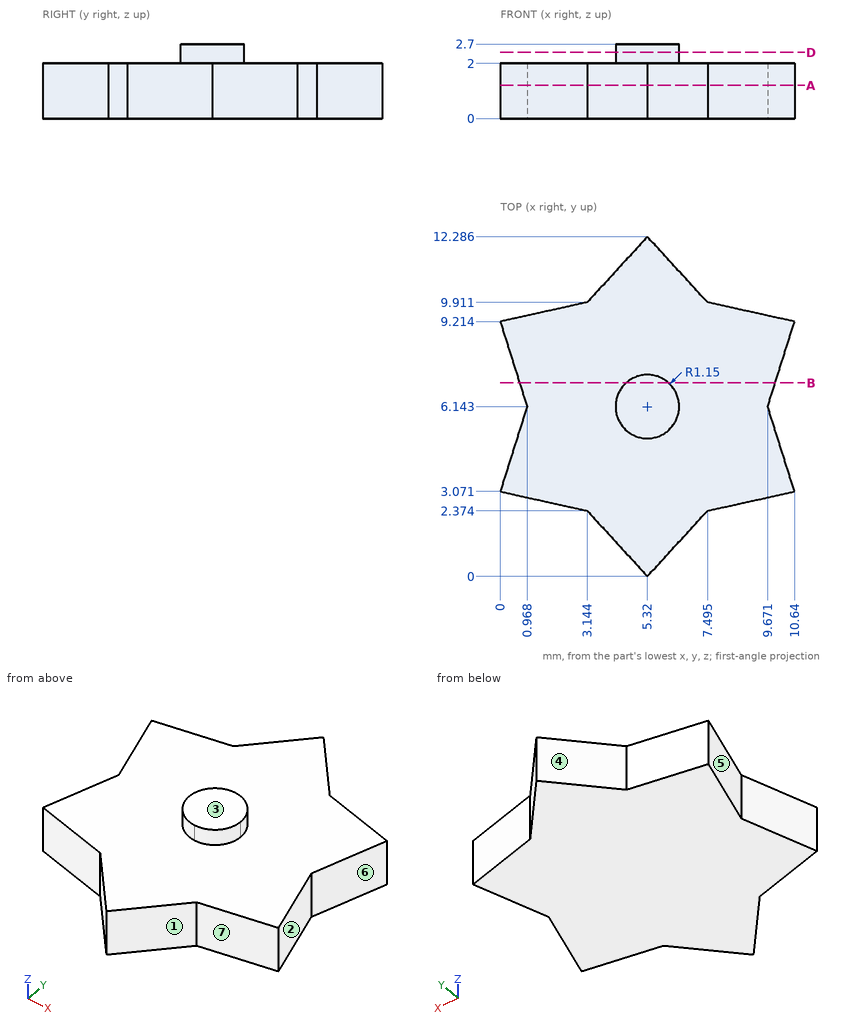
Part print with two shaded views. Sizes in mm from the minimum x, y, z corner. A direction names the side the tool comes from. Round coordinates to 2 decimals unless told otherwise and drop trailing zeros. Order: outer loops, then holes, each group sorted by start corner. A loop starts at its lowest first (then second) coordinate and runs counter-clockwise, first axis right, second up. Notation, with made-up numbers: M 40,-34.75 L 77,-34.75 A28 ccw 77,-1.75 Z; hole C 53,14 d7. An arc over 180 degrees is marked long. Answer in a Markdown table with one row per item. Add a question column.
Q1. Wall check: L1, parallel to Z at x = 5.75, y = 7.5; L2, parallel to X at y = 3.25, z = 1.2 (1 decimal); L3, parallel to Y at x = 6.25, z = 1.8 (1 decimal). Give the ranges that are in metal, low to high. Write a range as from..to.
Q2. Cut at B-B on y = 7. Give the cut face in (x, z).
Q3. Cut at D-D on z = 2.4. Give the cut face in (x, y).
Q4. 3-axis set-ups, long thin cutter, end or side, ignore diameter. For the marked faces 5, 6 and 7: which of +Z, -Z, +X, -X, +Y, -Y reach the whole face in a straight line?
Q5. Cut at A-A on z = 1.2. Give the cut face in (x, y) (1 decimal).
Q6. Mould opens along Y. For the marked faces 1, 2, 3 and 4 say: +Y half, -Y half, draft (parallel to the pull), parting line (faces both ways), or undercut.
Q7. Pin check, flat tip, straight feed: pin 1 (4 mm diameter, centred on x = 2, y = 4.5, fed in from +Z). Stop position of the tip, or through.
Established:
| question | item | result |
|---|---|---|
| 1 | L1 | z = 0..2 |
| 1 | L2 | x = 0.1..10.6 |
| 1 | L3 | y = 1..11.3 |
| 2 | outline | M 0.7,0 L 9.94,0 L 9.94,2 L 6.09,2 L 6.09,2.7 L 4.55,2.7 L 4.55,2 L 0.7,2 Z |
| 3 | outline | C 5.32,6.14 d2.3 |
| 4 | face 5 | +Z, -Z, -X |
| 4 | face 6 | +Z, -Z, +X |
| 4 | face 7 | +Z, -Z, +X, -Y |
| 5 | outline | M 0,3.1 L 3.1,2.4 L 5.3,0 L 7.5,2.4 L 10.6,3.1 L 9.7,6.1 L 10.6,9.2 L 7.5,9.9 L 5.3,12.3 L 3.1,9.9 L 0,9.2 L 1,6.1 Z |
| 6 | face 1 | -Y half |
| 6 | face 2 | undercut |
| 6 | face 3 | draft |
| 6 | face 4 | +Y half |
| 7 | pin 1 | stops at z = 2 |
